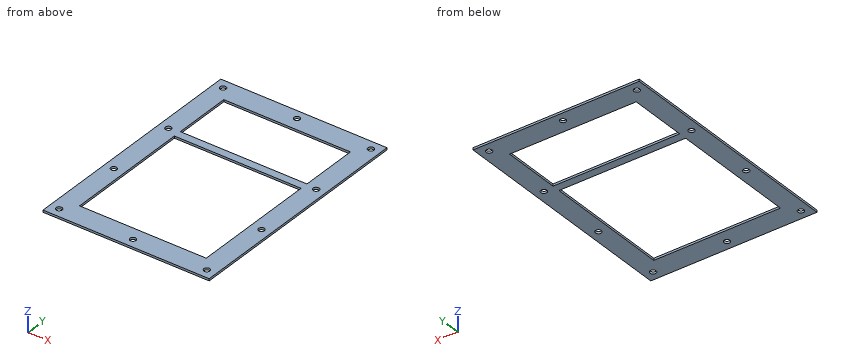
```python
from build123d import *

# Parameters (mm, degrees)
F0_W     = 63
F0_H     = 90
F1_DEPTH = 0.8
F3_R     = 1.1303
F4_DEPTH = 25
F5_W     = 48
F5_H     = 22
F5_H_2   = 48
F6_DEPTH = 25


with BuildPart() as f1:
    # F0 (on Top) → F1 (new body)
    with BuildSketch(Plane.XY):
        Rectangle(F0_W, F0_H)
    extrude(amount=F1_DEPTH)

    # F3 (on face) → F4 (cut)
    with BuildSketch(Plane.XY.offset(0.8)):
        with Locations((-28, 41.5)):
            Circle(F3_R)
        with Locations((-28, -41.5)):
            Circle(F3_R)
        with Locations((28, -41.5)):
            Circle(F3_R)
        with Locations((28, 41.5)):
            Circle(F3_R)
        with Locations((0, 41.5)):
            Circle(F3_R)
        with Locations((0, -41.5)):
            Circle(F3_R)
        with Locations((-28, 13.833333)):
            Circle(F3_R)
        with Locations((-28, -13.833333)):
            Circle(F3_R)
        with Locations((28, 13.833333)):
            Circle(F3_R)
        with Locations((28, -13.833333)):
            Circle(F3_R)
    extrude(amount=-F4_DEPTH, mode=Mode.SUBTRACT)

    # F5 (on face) → F6 (cut)
    with BuildSketch(Plane.XY.offset(0.8)):
        with Locations((0, 25.5)):
            Rectangle(F5_W, F5_H)
        with Locations((0, -12.5)):
            Rectangle(F5_W, F5_H_2)
    extrude(amount=-F6_DEPTH, mode=Mode.SUBTRACT)


solid = f1.part
```
Here's how the part is built. I have some questions about the finished solid (model axes, mm). Give positions to 0.01 mm unless a question says otherwise; leave off trailing zeros. Write each loop counter-clockwise with the first axis right and the second up, starting at its lowest first coordinate (ties: lowest second). Pieces come first, ordered by that corner, then holes.
(1) If I drill on L1, parallel to Y at x = 28, z = 0.4; L2, parallel to Y at x = -19.5, z = 0.35; L3, parallel to Y at x = 0, z = 0.35, over which ranges is the centre line in solid material (lowest first)?
Output values:
L1: y = -45 to -42.63, -40.37 to -14.96, -12.7 to 12.7, 14.96 to 40.37, 42.63 to 45
L2: y = -45 to -36.5, 11.5 to 14.5, 36.5 to 45
L3: y = -45 to -42.63, -40.37 to -36.5, 11.5 to 14.5, 36.5 to 40.37, 42.63 to 45
(2) Imagine slicing it at A-A, the plane x = 0. Write out the boundary of the cut face in (y, z), and give its area (3 significant figures).
Output values:
outline: (-45, 0) - (-42.63, 0) - (-42.63, 0.8) - (-45, 0.8) - close; (-40.37, 0) - (-36.5, 0) - (-36.5, 0.8) - (-40.37, 0.8) - close; (11.5, 0) - (14.5, 0) - (14.5, 0.8) - (11.5, 0.8) - close; (36.5, 0) - (40.37, 0) - (40.37, 0.8) - (36.5, 0.8) - close; (42.63, 0) - (45, 0) - (45, 0.8) - (42.63, 0.8) - close
area: 12.4 mm2
(3) Imagine slicing it at C-C, the plane x = 14. Write out the boundary of the cut face in (y, z), and give its area (3 significant figures).
Output values:
outline: (-45, 0) - (-36.5, 0) - (-36.5, 0.8) - (-45, 0.8) - close; (11.5, 0) - (14.5, 0) - (14.5, 0.8) - (11.5, 0.8) - close; (36.5, 0) - (45, 0) - (45, 0.8) - (36.5, 0.8) - close
area: 16.0 mm2
(4) Imagine slicing it at B-B, the plane y = 41.5. Write out the boundary of the cut face in (x, z), and give its area (3 significant figures).
Output values:
outline: (-31.5, 0) - (-29.13, 0) - (-29.13, 0.8) - (-31.5, 0.8) - close; (-26.87, 0) - (-1.13, 0) - (-1.13, 0.8) - (-26.87, 0.8) - close; (1.13, 0) - (26.87, 0) - (26.87, 0.8) - (1.13, 0.8) - close; (29.13, 0) - (31.5, 0) - (31.5, 0.8) - (29.13, 0.8) - close
area: 45.0 mm2
(5) Imagine slicing it at D-D, the plane y = 25. Write out the boundary of the cut face in (x, z).
Output values:
outline: (-31.5, 0) - (-24, 0) - (-24, 0.8) - (-31.5, 0.8) - close; (24, 0) - (31.5, 0) - (31.5, 0.8) - (24, 0.8) - close
